Check sheet for the modelled part. Datum: model origin and axes. Units: mm. A direction names the side the tool comes from. Coordinates: 2 decimals unless noted, no trailing zeros. Loops run counter-clockwise (first coordinate to the right, second up) from the corner with the lowest first, then second, coordinate; pieces in that order, holes last. Notation, with made-up numbers: M 42,18 L 75,18 A28 ccw 75,37 Z; hole C 22,14 d1. An arc over 180 degrees is marked long. Return JSON: item names as keys, results as strings.
from build123d import *

# Parameters (mm, degrees)
F5_DEPTH      = 0.1524
F6_COUNT      = 4
F8_DEPTH      = 3.3506944444
F10_DEPTH     = 12.0833333333
F11_T4_ANGLE  = 55.3885988596
F11_S5_R      = 0.0834798304
F11_T6_DEPTH  = 2
F11_T10_ANGLE = 55.3885988596
F11_S11_R     = 0.0834798304
F11_T12_DEPTH = 2
F11_T16_ANGLE = 55.3885988596
F11_S17_R     = 0.0833333333
F11_T18_DEPTH = 2


# Not quite as in the source:
# - a fillet or chamfer that OpenCascade refuses, or shapes differently, is made with other operations: its cross-section is extruded or revolved along the edge and cut away or added


with BuildPart() as f1:
    # F0 (on Front) → F1 (revolve)
    with BuildSketch(Plane.XZ):
        with BuildLine():
            Line((0, 25.4166666667), (0, 0))
            Line((0, 0), (0.7048611111, 0))
            Line((0.7048611111, 0), (0.7048611111, 21.8958333333))
            ThreePointArc((0.7048611111, 21.8958333333), (0.5269147233, 23.6911812486), (0, 25.4166666667))
        make_face()
    revolve(axis=Axis((0, 0, 12.7083333333), (0, 0, 1)))

    # F2 (on Front) → F3 (revolve, cut)
    with BuildSketch(Plane.XZ):
        Polygon((0.7048611111, 1.5625), (0.5729166667, 0), (0.7048611111, 0), (1.5729166667, 0), (1.5729166667, 1.5625), align=None)
    revolve(axis=Axis((0, 0, 0), (0, 0, 1)), mode=Mode.SUBTRACT)

    # F4 (on Front) → F5 (join, symmetric)
    with BuildSketch(Plane.XZ):
        Polygon((0.7048611111, 14.4444444444), (-0.7048611111, 14.4444444444), (-0.9131944444, 14.4444444444), (-3.5498263889, 11.6464416667), (-3.5498263889, 11.0214416667), (-0.7048611111, 11.0214416667), (0.7048611111, 11.0214416667), (3.5498263889, 11.0214416667), (3.5498263889, 11.6464416667), (0.9131944444, 14.4444444444), align=None)
        Polygon((2.8125, 0), (0.7048611111, 3.2631944444), (-0.7048611111, 3.2631944444), (-2.8125, 0), (-0.1651, 0), (0.1651, 0), align=None)
    extrude(amount=F5_DEPTH, both=True)

    # F6: F1 ×4 about axis
    f6_axis = Axis((0, 0, 0), (0, 0, 1))


with BuildPart() as f1_1:
    add(f1.part)
    for i in range(1, F6_COUNT):
        add(f1.part.rotate(f6_axis, i * 360 / F6_COUNT))

    # F7 (on face) → F8 (join, symmetric)
    with BuildSketch(Plane.XY.offset(14.4444444444)):
        with BuildLine():
            ThreePointArc((-0.5538420942, -0.435990964), (-0.5574412256, -0.5574412256), (-0.435990964, -0.5538420942))
            ThreePointArc((-0.435990964, -0.5538420942), (-0.4984120715, -0.4984120715), (-0.5538420942, -0.435990964))
        make_face()
        with BuildLine():
            ThreePointArc((-0.5538420942, -0.435990964), (-0.4984120715, -0.4984120715), (-0.435990964, -0.5538420942))
            Line((-0.435990964, -0.5538420942), (-0.3224915619, -0.4403426921))
            Line((-0.3224915619, -0.4403426921), (-0.4403426921, -0.3224915619))
            Line((-0.4403426921, -0.3224915619), (-0.5538420942, -0.435990964))
        make_face()
    extrude(amount=F8_DEPTH, both=True)

    # F9 (on face) → F10 (join)
    with BuildSketch(Plane(origin=(0, 0, 0), x_dir=(1, 0, 0), z_dir=(0, 0, -1))):
        with BuildLine():
            ThreePointArc((0.435990964, 0.5538420942), (0.4984120715, 0.4984120715), (0.5538420942, 0.435990964))
            ThreePointArc((0.5538420942, 0.435990964), (0.5538420942, 0.5538420942), (0.435990964, 0.5538420942))
        make_face()
        with BuildLine():
            ThreePointArc((0.3418792892, 0.4597304194), (0.4051132601, 0.4051132601), (0.4597304194, 0.3418792892))
            Line((0.4597304194, 0.3418792892), (0.5538420942, 0.435990964))
            ThreePointArc((0.5538420942, 0.435990964), (0.4984120715, 0.4984120715), (0.435990964, 0.5538420942))
            Line((0.435990964, 0.5538420942), (0.3418792892, 0.4597304194))
        make_face()
    extrude(amount=-F10_DEPTH)

    # F11: chamfer of 0.1 on 3 edges, made by hand


with BuildPart() as f11_tool2:
    # F11_s3 → F11_t4 (revolve)
    with BuildSketch(Plane(origin=(0, 0, 0), x_dir=(0, 0, 1), z_dir=(-0.2974698653, 0.9547312078, 0))):
        Polygon((17.8951388889, -0.7048611111), (17.7951388889, -0.8048611111), (17.7951388889, -0.7048611111), align=None)
    revolve(axis=Axis((0, 0, 17.7951388889), (0, 0, 1)), revolution_arc=F11_T4_ANGLE)

    # F11_s5 → F11_t6 (intersect, symmetric)
    with BuildSketch(Plane.XY.offset(17.8)):
        with Locations((-0.4984120715, -0.4984120715)):
            Circle(F11_S5_R)
    extrude(amount=F11_T6_DEPTH, both=True, mode=Mode.INTERSECT)


with BuildPart() as f1_2:
    add(f1_1.part)

    # F11_t1: union F11_tool2
    add(f11_tool2.part)


with BuildPart() as f11_tool8:
    # F11_s9 → F11_t10 (revolve)
    with BuildSketch(Plane(origin=(0, 0, 0), x_dir=(0, 0, 1), z_dir=(-0.2974698653, 0.9547312078, 0))):
        Polygon((10.99375, -0.7048611111), (11.09375, -0.8048611111), (11.09375, -0.7048611111), align=None)
    revolve(axis=Axis((0, 0, 11.09375), (0, 0, 1)), revolution_arc=F11_T10_ANGLE)

    # F11_s11 → F11_t12 (intersect, symmetric)
    with BuildSketch(Plane.XY.offset(11)):
        with Locations((-0.4984120715, -0.4984120715)):
            Circle(F11_S11_R)
    extrude(amount=F11_T12_DEPTH, both=True, mode=Mode.INTERSECT)


with BuildPart() as f1_3:
    add(f1_2.part)

    # F11_t7: union F11_tool8
    add(f11_tool8.part)


with BuildPart() as f11_tool14:
    # F11_s15 → F11_t16 (revolve)
    with BuildSketch(Plane(origin=(0, 0, 0), x_dir=(0, 0, 1), z_dir=(-0.9547312078, -0.2974698653, 0))):
        Polygon((12.1833333333, -0.7048611111), (12.0833333333, -0.8048611111), (12.0833333333, -0.7048611111), align=None)
    revolve(axis=Axis((0, 0, 12.0833333333), (0, 0, 1)), revolution_arc=F11_T16_ANGLE)

    # F11_s17 → F11_t18 (intersect, symmetric)
    with BuildSketch(Plane.XY.offset(12.1)):
        with Locations((0.4949165291, -0.4949165291)):
            Circle(F11_S17_R)
    extrude(amount=F11_T18_DEPTH, both=True, mode=Mode.INTERSECT)


with BuildPart() as f1_4:
    add(f1_3.part)

    # F11_t13: union F11_tool14
    add(f11_tool14.part)


solid = f1_4.part
1) Draft check along Z on faces 4 (the face through (-1.744, -0.002, 1.654)), 5 (the face through (2, 0.152, 12)), 6 (the face through (0, -2.21, 13.07)). Enter one of: +Z half, -Z half, draft (parallel to the pull), parting line (faces both ways), or undercut.
Answers:
{"face 4": "undercut", "face 5": "draft", "face 6": "+Z half"}
2) Section check B-B on x = -1.25. Record the cut outline in (y, z).
Answers:
{"outline": "M -0.15,0 L 0.15,0 L 0.15,2.42 L -0.15,2.42 Z; M -0.15,11.02 L 0.15,11.02 L 0.15,14.09 L -0.15,14.09 Z"}
3) Section check A-A on y = 2.5. Record the cut outline in (x, z), then the cut area to 3 significant figures.
Answers:
{"outline": "M -0.15,0 L 0.15,0 L 0.15,0.48 L -0.15,0.48 Z; M -0.15,11.02 L 0.15,11.02 L 0.15,12.76 L -0.15,12.76 Z", "area": "0.678 mm²"}
4) Set-up check for faces 1 (the face through (0.152, 2, 12)), 2 (the face through (-0.152, 2, 12)), 3 (the face through (2, -0.152, 12)): record each of +Z, -Z, +X, -X, +Y, -Y from which the full face is reachable in a straight line by a thin tool's end or side.
Answers:
{"face 1": "+Z, -Z, +X, +Y", "face 2": "+Z, -Z, -X, +Y", "face 3": "+Z, -Z, +X, -Y"}
5) Section check D-D on z = 6.25. Record the cut outline in (x, y), then the cut area to 3 significant figures.
Answers:
{"outline": "M 0.44,-0.55 A0.08 ccw 0.55,-0.44 A0.7 ccw long Z", "area": "1.57 mm²"}
6) Section check C-C on z = 20. Record the cut outline in (x, y), then the cut area to 3 significant figures.
Answers:
{"outline": "C 0,0 d1.41", "area": "1.56 mm²"}
7) Scan lines: line 1 along Z through (x, y) = (0, 1.25); line 2 along Y through (x, z) = (0, 18.75); line 3 along Y through (x, z) = (-0.5, 1). Record each from-to range of solid material in increasing order. Write a range as [from, to].
Answers:
{"line 1": "[0, 2.42], [11.02, 14.09]", "line 2": "[-0.7, 0.7]", "line 3": "[-0.43, 0.43]"}
8) Go/stop test with flat-tipped pins: pin 1 Ø1.8 at (x, z) = (2, 1.5) entering from -Y; pin 2 Ø4 at (y, z) = (0.5, 19.5) entering from -X; pin 3 Ø4 at (x, z) = (0.5, 16.5) entering from -Y. Record where each tip stops, or that it passes through.
Answers:
{"pin 1": "y = -0.15", "pin 2": "x = -0.7", "pin 3": "y = -0.7"}
